```python
from build123d import *

# Parameters (mm, degrees)
SKETCH1_W           = 37
SKETCH1_H           = 8
BOSS_EXTRUDE1_DEPTH = 2
SKETCH2_R           = 1
CUT_EXTRUDE1_DEPTH  = 3
SKETCH3_W           = 2.5
SKETCH3_H           = 4
SKETCH3_H_2         = 1
BOSS_EXTRUDE2_DEPTH = 3


with BuildPart() as part:
    # Sketch1 → Boss-Extrude1 (new body)
    with BuildSketch(Plane(origin=(0, 0, 0), x_dir=(1, 0, 0), z_dir=(0, 1, 0))):
        Rectangle(SKETCH1_W, SKETCH1_H)
    extrude(amount=BOSS_EXTRUDE1_DEPTH)

    # Sketch2 → Cut-Extrude1 (cut, through all)
    with BuildSketch(Plane(origin=(0, 2, 0), x_dir=(1, 0, 0), z_dir=(0, 1, 0))):
        with Locations((-0.58, -0.8)):
            Circle(SKETCH2_R)
    extrude(amount=-CUT_EXTRUDE1_DEPTH, mode=Mode.SUBTRACT)

    # Sketch3 → Boss-Extrude2 (add)
    with BuildSketch(Plane.XZ):
        with Locations((17.25, 0)):
            Rectangle(SKETCH3_W, SKETCH3_H)
        with Locations((17.25, -3.5)):
            Rectangle(SKETCH3_W, SKETCH3_H_2)
        with Locations((-17.25, -3.5)):
            Rectangle(SKETCH3_W, SKETCH3_H_2)
        with Locations((-17.25, 0)):
            Rectangle(SKETCH3_W, SKETCH3_H)
    extrude(amount=BOSS_EXTRUDE2_DEPTH)


solid = part.part
```
For this review, take the finished solid that the model builds, in its own axes (mm). A direction names the side the tool comes from. Round coordinates to 2 decimals unless told otherwise and drop trailing zeros. Write each loop counter-clockwise with the first axis right and the second up, starting at its lowest first coordinate (ties: lowest second). Pieces come first, ordered by that corner, then holes. Notation, with made-up numbers: (82.25, -16.75) - (106.25, -16.75) arc R37 cw to (106.25, 21.25) - close; hole circle Ø1 at (32.5, -11). An arc over 180 degrees is marked (long way). Answer as CSV lines item,"result". Start each with the question number.
(1) For line 1 (Z direction, x = -0.58, y = 0.5); line 2 (X direction, y = 0.55, z = 0.8); line 3 (X direction, y = -2.45, z = -3.5), list the stretches that pass through material, from the lowest coordinate up.
(2) Mouldability with a two-part tool opening along Z and no side actions: class faces 6 (the flat face through (0, 1, -4)), 7 (the flat face through (17, -1, -3)), 8 (the flat face through (0, 2, -1)), 9 (the flat face through (0, 1, 4)) as +Z half, -Z half, draft (parallel to the pull), parting line (faces both ways), or undercut.
(3) Add section A-A, the plane x = -0.58. State the section outline as (y, z) points.
(4) Add section C-C, the plane y = -2.35. State the section outline as (x, z) points, plus the area to 3 significant figures.
(5) For pin 1 (2 mm diameter, centred on x = 17.5, y = -2, fed in from +Z), flat-tipped, find the tip position at first contact; note if it passes through.
(6) Add section B-B, the plane z = 0.8. State the section outline as (x, y) points, plus the area to 3 significant figures.
(7) Machinability: for faces 1 (the flat face through (16, -1, 0)), 2 (the flat face through (17, -1, -2)), 3 (the flat face through (18.5, 0, 0)), 4 (the flat face through (-18.5, -1, 0)), 5 (the flat face through (-17, -1, 2)), which of the approach directions +Z, -Z, +X, -X, +Y, -Y give a long, thin tool a straight path to every point of the face, cutting with its end or side? Answer none if there is none.
From the geometry:
1,line 1,"z = -4 to -0.2, 1.8 to 4"
1,line 2,"x = -18.5 to -1.58, 0.42 to 18.5"
1,line 3,"x = -18.5 to -16, 16 to 18.5"
2,face 6,"-Z half"
2,face 7,"undercut"
2,face 8,"draft"
2,face 9,"+Z half"
3,outline,"(0, -4) - (2, -4) - (2, -0.2) - (0, -0.2) - close; (0, 1.8) - (2, 1.8) - (2, 4) - (0, 4) - close"
4,outline,"(-18.5, -4) - (-16, -4) - (-16, -3) - (-18.5, -3) - close; (-18.5, -2) - (-16, -2) - (-16, 2) - (-18.5, 2) - close; (16, -4) - (18.5, -4) - (18.5, -3) - (16, -3) - close; (16, -2) - (18.5, -2) - (18.5, 2) - (16, 2) - close"
4,area,"25.0 mm²"
5,pin 1,"stops at z = 2"
6,outline,"(-18.5, -3) - (-16, -3) - (-16, 0) - (-1.58, 0) - (-1.58, 2) - (-18.5, 2) - close; (0.42, 0) - (16, 0) - (16, -3) - (18.5, -3) - (18.5, 2) - (0.42, 2) - close"
6,area,"85.0 mm²"
7,face 1,"+Z, -Z, -Y"
7,face 2,"+X, -X, -Y"
7,face 3,"+Z, -Z, +X, +Y, -Y"
7,face 4,"+Z, -Z, -X, +Y, -Y"
7,face 5,"+Z, +X, -X, -Y"
